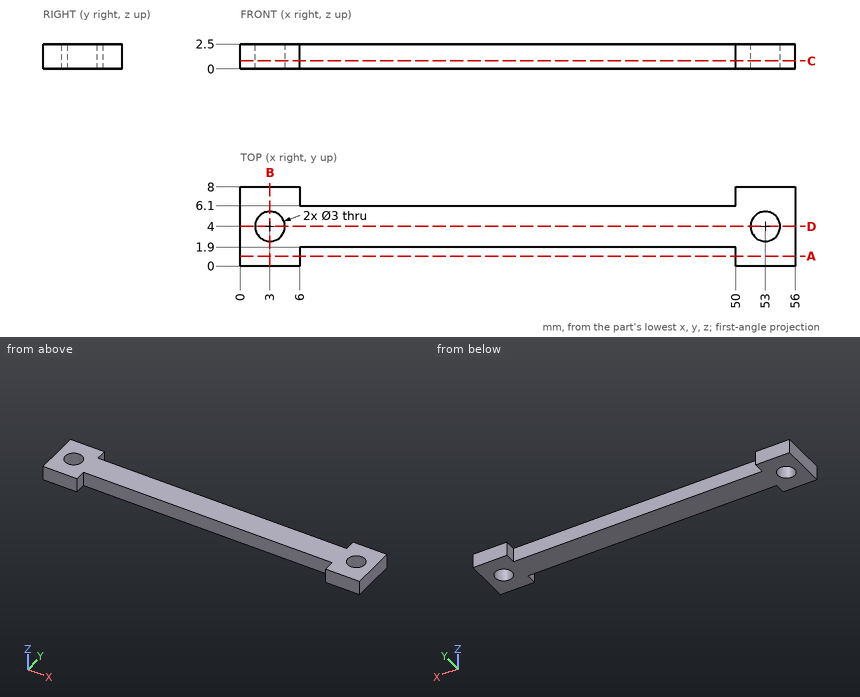
Check sheet for the drawn part. Datum: minimum x, y, z corner. Units: mm. Give positions to 0.01 mm unless a question says otherwise; leave off trailing zeros. Order: outer loops, then holes, each group sorted by start corner. A loop starts at its lowest first (then second) coordinate and runs counter-clockwise, first axis right, second up. Notation, with made-up numbers: (-32.5, -3.75) -> (15.5, -3.75) arc R15 ccw to (15.5, 2.25) -> close; hole circle Ø11 at (72, 36.5). An arc over 180 degrees is marked (long way). Answer as CSV lines item,"result".
Q1. Sectioned sample at A-A on y = 1. Record the cut outline in (x, z), plus the area to 3 significant figures.
Solutions:
outline,"(0, 0) -> (6, 0) -> (6, 2.5) -> (0, 2.5) -> close; (50, 0) -> (56, 0) -> (56, 2.5) -> (50, 2.5) -> close"
area,"30.0 mm²"
Q2. Scan lines: probe 1 along Y at (x, z) = (3, 1.3); probe 2 along X at (y, z) = (2.75, 0.9); probe 3 along X at (y, z) = (6.5, 0.4). Record each from-to range of solid material in increasing order.
Solutions:
probe 1,"y = 0 to 2.5, 5.5 to 8"
probe 2,"x = 0 to 2.17, 3.83 to 52.17, 53.83 to 56"
probe 3,"x = 0 to 6, 50 to 56"
Q3. Sectioned sample at C-C on z = 0.8. Record the cut outline in (x, y).
Solutions:
outline,"(0, 0) -> (6, 0) -> (6, 1.9) -> (50, 1.9) -> (50, 0) -> (56, 0) -> (56, 8) -> (50, 8) -> (50, 6.1) -> (6, 6.1) -> (6, 8) -> (0, 8) -> close; hole circle Ø3 at (3, 4); hole circle Ø3 at (53, 4)"
Q4. Sectioned sample at B-B on x = 3. Record the cut outline in (y, z), plus the area to 3 significant figures.
Solutions:
outline,"(0, 0) -> (2.5, 0) -> (2.5, 2.5) -> (0, 2.5) -> close; (5.5, 0) -> (8, 0) -> (8, 2.5) -> (5.5, 2.5) -> close"
area,"12.5 mm²"
Q5. Depth check by flat-ended pin: pin 1 (1 mm diameter, centred on x = 43, z = 1, fed in from -Y); pin 2 (2 mm diameter, centred on x = 38, y = 5.5, fed in from -Z). Enter the tip coordinate at first touch or a pass-through.
Solutions:
pin 1,"stops at y = 1.9"
pin 2,"stops at z = 0"
Q6. Sectioned sample at D-D on y = 4. Record the cut outline in (x, z).
Solutions:
outline,"(0, 0) -> (1.5, 0) -> (1.5, 2.5) -> (0, 2.5) -> close; (4.5, 0) -> (51.5, 0) -> (51.5, 2.5) -> (4.5, 2.5) -> close; (54.5, 0) -> (56, 0) -> (56, 2.5) -> (54.5, 2.5) -> close"
